Geometry check sheet. Reference: the model listing, model coordinates, mm. A direction names the side the tool comes from. Coordinates: 2 decimals unless noted, no trailing zeros. Loops run counter-clockwise (first coordinate to the right, second up) from the corner with the lowest first, then second, coordinate; pieces in that order, holes last.
from build123d import *

# Parameters (mm, degrees)
SKETCH1_R           = 1.5
BOSS_EXTRUDE1_DEPTH = 6
FILLET1_R           = 9


with BuildPart() as part:
    # Sketch1 → Boss-Extrude1 (new body)
    with BuildSketch(Plane(origin=(0, 0, 0), x_dir=(1, 0, 0), z_dir=(0, 1, 0))):
        Polygon((-17.7, 15), (0, 15), (0, -15), (-3.3, -15), (-3.3, -9), (-1.9, -9), (-1.9, -6.8), (-3.3, -6.8), (-3.3, -4), (-6.3, -4), (-6.3, -6.8), (-7.7, -6.8), (-7.7, -9), (-6.3, -9), (-6.3, -15), (-17.7, -15), align=None)
        with Locations(Location((-8.7, 6, 0), (0, 0, 270))):
            Circle(SKETCH1_R, mode=Mode.SUBTRACT)
    extrude(amount=BOSS_EXTRUDE1_DEPTH)

    # Mirror1: part across plane


with BuildPart() as part_1:
    add(part.part)
    add(part.part.mirror(Plane(origin=(0, 6, -15), x_dir=(0, 0, 1), z_dir=(-1, 0, 0))))

    # Fillet1
    fillet1_edges = [part_1.edges().sort_by_distance(p)[0] for p in [
        (-17.7, 3, -15),
        (17.7, 3, -15),
    ]]
    fillet(fillet1_edges, radius=FILLET1_R)


solid = part_1.part
1) Section check A-A on z = 4.5. Record the cut outline in (x, y).
Data:
outline: (-17.7, 0) - (-6.3, 0) - (-6.3, 6) - (-17.7, 6) - close; (-3.3, 0) - (3.3, 0) - (3.3, 6) - (-3.3, 6) - close; (6.3, 0) - (17.7, 0) - (17.7, 6) - (6.3, 6) - close
2) Section check C-C on x = 5.5. Record the cut outline in (y, z).
Data:
outline: (0, -15) - (6, -15) - (6, 4) - (0, 4) - close
3) Mould release check, pull along Z, two halves, no side actions. Record for faces 4 (the flat face through (7, 3, 6.8)), 5 (the flat face through (0, 3, -15)), 6 (the flat face through (12, 3, 15)), 7 (the flat face through (6.3, 3, 5)): +Z half, -Z half, draft (parallel to the pull), parting line (faces both ways), or undercut.
Data:
face 4: undercut
face 5: -Z half
face 6: +Z half
face 7: draft
4) Section check B-B on y = 4.2. Count the separate pieces of the cut face and the enclosed holes in it, and give its area (3 significant figures).
Data:
separate pieces: 1
enclosed holes: 2
area: 935 mm2
5) Access from +Z, -Z, +X, -X, +Y, -Y to the whole of each face (thin tool, end or side, straight path). Record for faces 1 (the flat face through (-17.7, 3, 5)), 2 (the flat face through (-6.3, 3, 12)), 3 (the flat face through (-7, 3, 9)).
Data:
face 1: +Z, -Z, -X, +Y, -Y
face 2: +Z, +Y, -Y
face 3: +Y, -Y
6) Material ranges on probe 1 along X at (y, z) = (4, -6); probe 2 along X at (y, z) = (0.35, 11.75); probe 3 along Z at (x, y) = (6, 4.1), recorded low to high.
Data:
probe 1: x = -17.7 to -10.2, -7.2 to 7.2, 10.2 to 17.7
probe 2: x = -17.7 to -6.3, -3.3 to 3.3, 6.3 to 17.7
probe 3: z = -15 to 4
7) Depth check by flat-ended pin: pin 1 (2 mm diameter, centred on x = -14, y = 3.5, fed in from -Z); pin 2 (0.9 mm diameter, centred on x = -5, y = 2, fed in from +Z). Enter the tip coordinate at first touch or a pass-through.
Data:
pin 1: stops at z = -13.91
pin 2: stops at z = 4
8) Section check D-D on z = -5. Record the cut outline in (x, y).
Data:
outline: (-17.7, 0) - (-9.82, 0) - (-9.82, 6) - (-17.7, 6) - close; (-7.58, 0) - (7.58, 0) - (7.58, 6) - (-7.58, 6) - close; (9.82, 0) - (17.7, 0) - (17.7, 6) - (9.82, 6) - close
